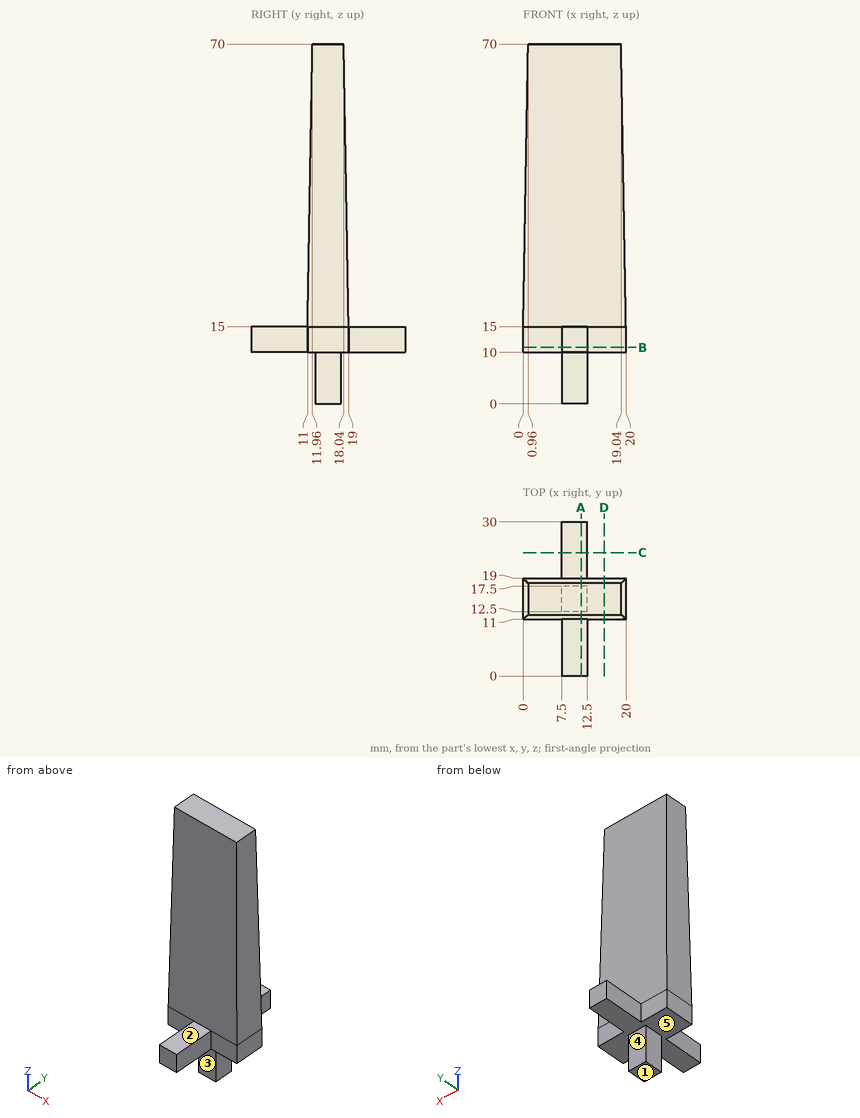
Here's the drawing with two shaded views (mm, measured from the low corner). I have some questions. A direction names the side the tool comes from. Give positions to 0.01 mm unless a question says otherwise; leave off trailing zeros. Write each loop counter-clockwise with the first axis right and the second up, starting at its lowest first coordinate (ties: lowest second). Pieces come first, ordered by that corner, then holes. Notation, with made-up numbers: (30, 50) -> (43, 50) arc R17 ccw to (43, 76) -> close; hole circle Ø2 at (-36.75, -14.5). An arc over 180 degrees is marked (long way). One line per item, written item: value.
Q1. Imagine slicing it at C-C on y = 24. Please give me the cut outline in (x, z).
Results found:
outline: (7.5, 10) -> (12.5, 10) -> (12.5, 15) -> (7.5, 15) -> close
Q2. Imagine slicing it at D-D on x = 15.75. Please give me the cut outline in (y, z).
Results found:
outline: (11, 10) -> (19, 10) -> (19, 15) -> (18.04, 70) -> (11.96, 70) -> (11, 15) -> close
Q3. Please list where these lines run through material, in increasing order: line 1 (Z direction, x = 17, y = 18); line 2 (Z direction, x = 8.5, y = 23.25); line 3 (X direction, y = 21.5, z = 12.5). Write a range as [from, to].
Results found:
line 1: z = [10, 70]
line 2: z = [10, 15]
line 3: x = [7.5, 12.5]
Q4. We'd pull the mould along Y, two halves only. Please class the marked faces 3, 4 and 5: +Y half, -Y half, draft (parallel to the pull), parting line (faces both ways), or undercut.
Results found:
face 3: -Y half
face 4: +Y half
face 5: draft
Q5. Which directions (+Z, -Z, +X, -X, +Y, -Y) give clear straight access to the entire face, cutting with the end or side of a thin tool? Please do the marked faces 1 and 2.
Results found:
face 1: -Z, +X, -X, +Y, -Y
face 2: +Z, +X, -X, -Y
Q6. Imagine slicing it at B-B on z = 11. Please give me the cut outline in (x, y), and give its area (3 significant figures).
Results found:
outline: (0, 11) -> (7.5, 11) -> (7.5, 0) -> (12.5, 0) -> (12.5, 11) -> (20, 11) -> (20, 19) -> (12.5, 19) -> (12.5, 30) -> (7.5, 30) -> (7.5, 19) -> (0, 19) -> close
area: 270 mm^2
Q7. Imagine slicing it at A-A on x = 11.25. Please give me the cut outline in (y, z), and give its area (3 significant figures).
Results found:
outline: (0, 10) -> (12.5, 10) -> (12.5, 0) -> (17.5, 0) -> (17.5, 10) -> (30, 10) -> (30, 15) -> (19, 15) -> (18.04, 70) -> (11.96, 70) -> (11, 15) -> (0, 15) -> close
area: 587 mm^2
Q8. For P1, Ø3, axis at x = 15, y = 17.5, coming from the -Z side; P2, Ø5.5, axis at x = 2.5, z = 12.5, coming from the -Y side; P3, Ø1.5, axis at x = 16.5, z = 32.5, coming from the +Y side, each with a flat end and sliding along its axis, tell me the tip position at first contact or that it passes through.
Results found:
P1: stops at z = 10
P2: stops at y = 11
P3: stops at y = 18.71
